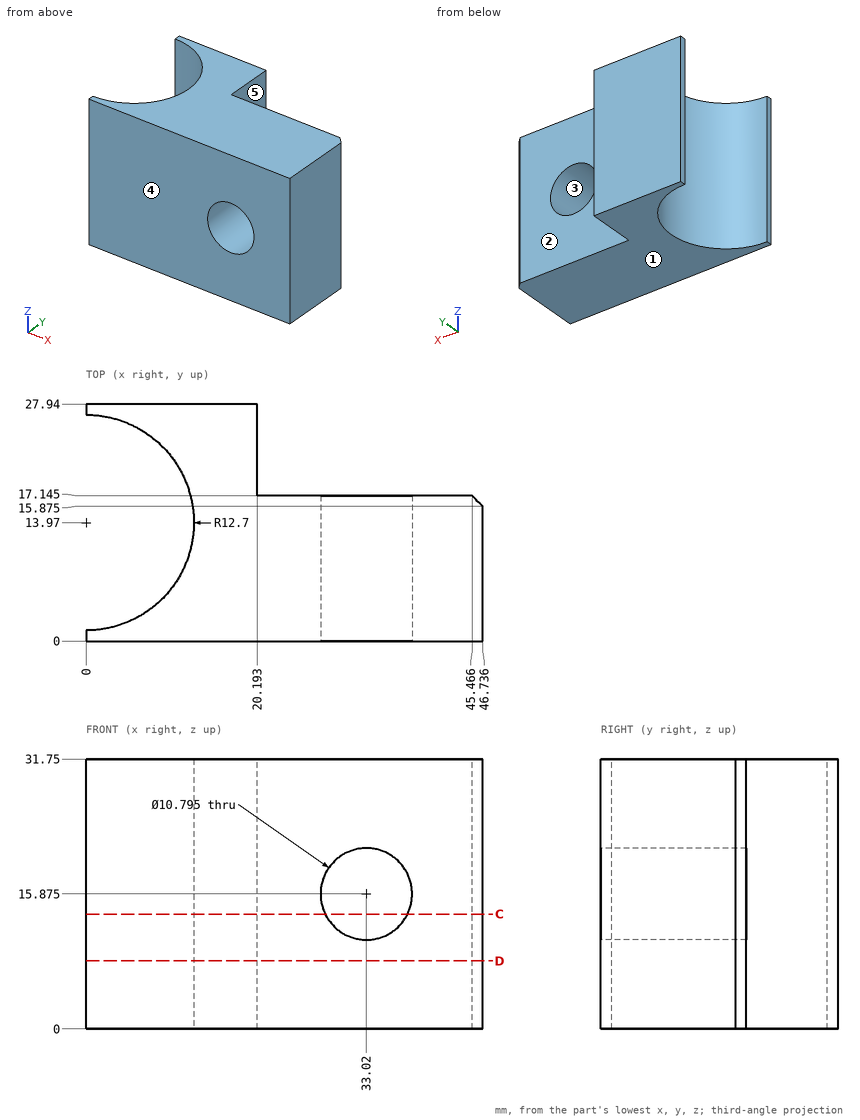
Print and shaded views of the part. All mm, measured from the part's lowest x, y and z. A direction names the side the tool comes from. Round coordinates to 2 decimals unless told otherwise and drop trailing zeros. Write each loop counter-clockwise with the first axis right and the second up, starting at its lowest first coordinate (ties: lowest second). Pieces come first, ordered by that corner, then holes. Notation, with made-up numbers: (25, 89.25) -> (69, 89.25) arc R28 cw to (69, 125.25) -> close; hole circle Ø3 at (75.25, 68). An arc over 180 degrees is marked (long way). Answer in a Markdown table with one row per item. Add a question column.
Item 1: Drill centre lines: line 1 (Z direction, x = 33.02, y = 6.5); line 2 (Y direction, x = 20.5, z = 21.5) (3 decimals); line 3 (Y direction, x = 4.5, z = 25). Where is each one in solid material? Low to high. Write a range as from..to.
Item 2: Saw through at C-C, the plane z = 13.5. Write the cut outline in (x, y) (3 decimals), then the cut area to 3 significant figures.
Item 3: Saw through at D-D, the plane z = 8. Write the cut outline in (x, y) (3 decimals).
Item 4: Mould opens along X. For the marked faces 3, 4 and 5 say: pulls with the +X half, pulls with the -X half, needs draft (parallel to the pull), parting line crosses it, or undercut.
Item 5: Drop flat-ended pins along their axis: pin 1 Ø8 at (y, z) = (20.5, 6) entering from +X; pin 2 Ø14 at (x, z) = (33.02, 15.875) entering from +Y (3 decimals); pin 3 Ø5.5 at (y, z) = (24.5, 16) entering from +X. Give the stop position or say it passes through.
Item 6: Which spindle directions (+Z, -Z, +X, -X, +Y, -Y) get a long thin tool onto all of the face, cutting with end or side? Do the marked faces 1 and 2. Say none if no direction does.
Findings below:
| question | item | result |
|---|---|---|
| 1 | line 1 | z = 0..10.48, 21.27..31.75 |
| 1 | line 2 | y = 0..17.145 |
| 1 | line 3 | y = 0..2.09, 25.85..27.94 |
| 2 | outline | (0, 0) -> (28.173, 0) -> (28.173, 17.145) -> (20.193, 17.145) -> (20.193, 27.94) -> (0, 27.94) -> (0, 26.67) arc R12.7 cw to (0, 1.27) -> close; (37.867, 0) -> (46.736, 0) -> (46.736, 15.875) -> (45.466, 17.145) -> (37.867, 17.145) -> close |
| 2 | area | 599 mm^2 |
| 3 | outline | (0, 0) -> (46.736, 0) -> (46.736, 15.875) -> (45.466, 17.145) -> (20.193, 17.145) -> (20.193, 27.94) -> (0, 27.94) -> (0, 26.67) arc R12.7 cw to (0, 1.27) -> close |
| 4 | face 3 | undercut |
| 4 | face 4 | needs draft |
| 4 | face 5 | pulls with the +X half |
| 5 | pin 1 | stops at x = 46.11 |
| 5 | pin 2 | stops at y = 17.145 |
| 5 | pin 3 | stops at x = 20.19 |
| 6 | face 1 | -Z, +X, -X, +Y, -Y |
| 6 | face 2 | +Z, -Z, +X, +Y |
